For this review, use the dimensioned drawing (mm, ordinates from the lowest corner) and the shaded views. Coordinates: 2 decimals unless noted, no trailing zeros. Loops run counter-clockwise (first coordinate to the right, second up) from the corner with the lowest first, then second, coordinate; pieces in that order, holes last. Notation, with made-up numbers: M -4,25 L 34,25 A36 ccw 34,63 Z; hole C 44,59.25 d9. An arc over 180 degrees is marked long. One line per item, written item: value.
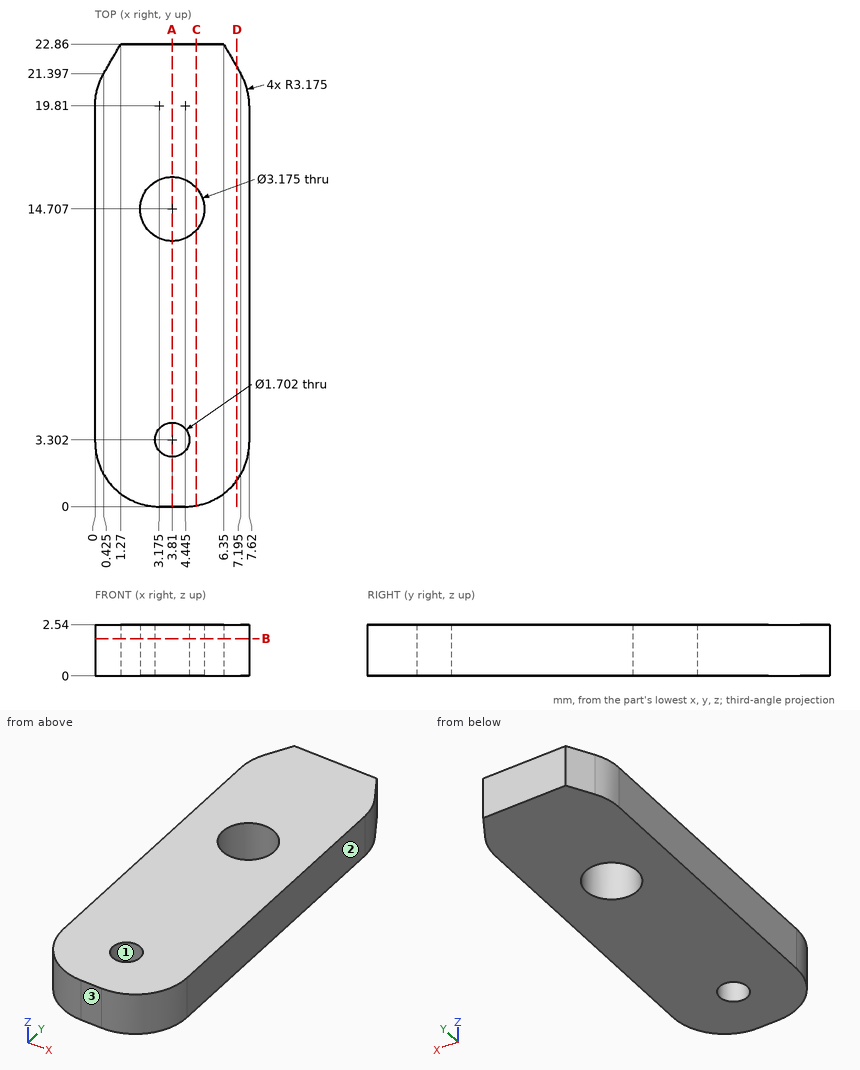
(1) We need section A-A on x = 3.81. State the section outline as (y, z) points.
Reply:
outline: M 0,0 L 2.45,0 L 2.45,2.54 L 0,2.54 Z; M 4.15,0 L 13.12,0 L 13.12,2.54 L 4.15,2.54 Z; M 16.29,0 L 22.86,0 L 22.86,2.54 L 16.29,2.54 Z
(2) We need section C-C on x = 5. State the section outline as (y, z) points (1 decimal).
Reply:
outline: M 0,0 L 13.7,0 L 13.7,2.5 L 0,2.5 Z; M 15.8,0 L 22.9,0 L 22.9,2.5 L 15.8,2.5 Z
(3) We need section D-D on x = 7. State the section outline as (y, z) points (1 decimal).
Reply:
outline: M 1.3,0 L 21.7,0 L 21.7,2.5 L 1.3,2.5 Z
(4) Mouldability with a two-part tool opening along Y and no side actions: class the marked faces 1, 2 and 3 as released by +Y, released by -Y, zero draft, split by the parting line, or undercut.
Reply:
face 1: undercut
face 2: zero draft
face 3: released by -Y
(5) To check wall thickness, follow line 1 along Y through (x, z) = (3.81, 0.6) (1 decimal); line 2 along Y through (x, z) = (4.5, 1.8) (1 decimal); line 3 along X through (y, z) = (15, 1.45). State the ranges of each line that lie inside material, in increasing order. Write a range as [from, to].
Reply:
line 1: y = [0, 2.5], [4.2, 13.1], [16.3, 22.9]
line 2: y = [0, 2.8], [3.8, 13.3], [16.1, 22.9]
line 3: x = [0, 2.25], [5.37, 7.62]
(6) We need section B-B on z = 1.85. State how many separate pieces and enclosed holes the cut face has, then the cut area to 3 significant figures.
Reply:
separate pieces: 1
enclosed holes: 2
area: 157 mm2
